from build123d import *

# Parameters (mm, degrees)
SKETCH1_W           = 35.8
SKETCH1_H           = 18.2
SKETCH1_R           = 1
SKETCH1_W_2         = 22.5
SKETCH1_H_2         = 12.2
BOSS_EXTRUDE1_DEPTH = 1.5
FILLET1_R           = 5


with BuildPart() as part:
    # Sketch1 → Boss-Extrude1 (new body, symmetric)
    with BuildSketch(Plane(origin=(0, 0, 0), x_dir=(1, 0, 0), z_dir=(0, 1, 0))):
        Rectangle(SKETCH1_W, SKETCH1_H)
        with Locations((-13.9, 0)):
            Circle(SKETCH1_R, mode=Mode.SUBTRACT)
        with Locations((13.9, 0)):
            Circle(SKETCH1_R, mode=Mode.SUBTRACT)
        Rectangle(SKETCH1_W_2, SKETCH1_H_2, mode=Mode.SUBTRACT)
    extrude(amount=BOSS_EXTRUDE1_DEPTH, both=True)

    # Fillet1
    fillet1_edges = [part.edges().sort_by_distance(p)[0] for p in [
        (-17.9, 0, -9.1),
        (17.9, 0, -9.1),
        (17.9, 0, 9.1),
        (-17.9, 0, 9.1),
    ]]
    fillet(fillet1_edges, radius=FILLET1_R)


solid = part.part
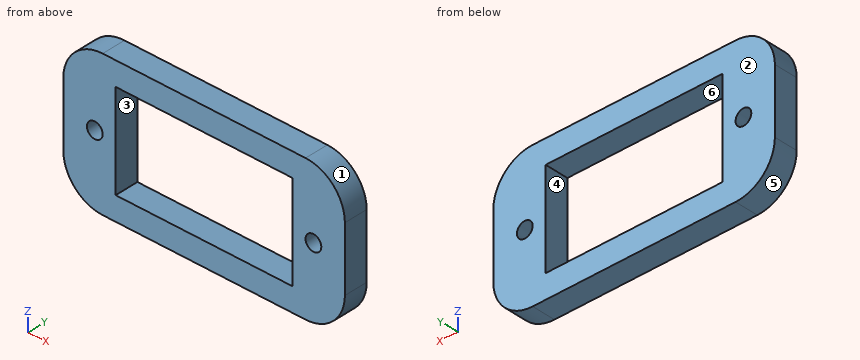
Could you check a few things on this model? Use its own coordinates, in mm. Face numbers are marked on the shaded views. A direction names the side the tool comes from. Coordinates: 2 decimals unless noted, no trailing zeros. Loops run counter-clockwise (first coordinate to the right, second up) from the corner with the lowest first, then second, coordinate; pieces in that order, holes last.
1. I need wall thicknesses on L1, parallel to X at y = -0.5, z = 0; L2, parallel to X at y = -0.65, z = 1.25; L3, parallel to Z at x = 0, y = -1.1. Which ranges of each line are inside material? Lowest first, please.
2. Imagine slicing it at B-B (z = 0). Please give me the cut outline in (x, y).
3. Imagine slicing it at D-D (z = -3). Please give me the cut outline in (x, y), and give its area (3 significant figures).
4. For P1, Ø4, axis at x = -6.5, z = -4.5, coming from the +Y side, with a flat end and sliding along its axis, tell me the tip position at first contact or that it passes through.
5. Imagine slicing it at C-C (y = 0.85). Please give me the cut outline in (x, z), and give its area (3 significant figures).
6. Imagine slicing it at A-A (x = 4). Please give me the cut outline in (y, z), and give its area (3 significant figures).
7. We'd pull the mould along Z, two halves only. Please class the marked faces 1, 2, 3 and 4: released by +Z, released by -Z, zero draft, split by the parting line, or undercut.
8. For the marked faces 5 and 6, which set-ups out of +Z, -Z, +X, -X, +Y, -Y let a thin tool reach every point of the face, with its end or its side?
Computed values:
1. L1: x = -17.9 to -14.9, -12.9 to -11.25, 11.25 to 12.9, 14.9 to 17.9
1. L2: x = -17.9 to -11.25, 11.25 to 17.9
1. L3: z = -9.1 to -6.1, 6.1 to 9.1
2. outline: (-17.9, -1.5) - (-14.9, -1.5) - (-14.9, 1.5) - (-17.9, 1.5) - close; (-12.9, -1.5) - (-11.25, -1.5) - (-11.25, 1.5) - (-12.9, 1.5) - close; (11.25, -1.5) - (12.9, -1.5) - (12.9, 1.5) - (11.25, 1.5) - close; (14.9, -1.5) - (17.9, -1.5) - (17.9, 1.5) - (14.9, 1.5) - close
3. outline: (-17.9, -1.5) - (-11.25, -1.5) - (-11.25, 1.5) - (-17.9, 1.5) - close; (11.25, -1.5) - (17.9, -1.5) - (17.9, 1.5) - (11.25, 1.5) - close
3. area: 39.9 mm2
4. P1: stops at y = 1.5
5. outline: (-17.9, -4.1) arc R5 ccw to (-12.9, -9.1) - (12.9, -9.1) arc R5 ccw to (17.9, -4.1) - (17.9, 4.1) arc R5 ccw to (12.9, 9.1) - (-12.9, 9.1) arc R5 ccw to (-17.9, 4.1) - close; hole circle Ø2 at (-13.9, 0); hole (-11.25, -6.1) - (11.25, -6.1) - (11.25, 6.1) - (-11.25, 6.1) - close; hole circle Ø2 at (13.9, 0)
5. area: 349 mm2
6. outline: (-1.5, -9.1) - (1.5, -9.1) - (1.5, -6.1) - (-1.5, -6.1) - close; (-1.5, 6.1) - (1.5, 6.1) - (1.5, 9.1) - (-1.5, 9.1) - close
6. area: 18.0 mm2
7. face 1: released by +Z
7. face 2: zero draft
7. face 3: undercut
7. face 4: undercut
8. face 5: -Z, -X, +Y, -Y
8. face 6: +Y, -Y
